from build123d import *

# Parameters (mm, degrees)
SKETCH1_R             = 45
SKETCH1_R_2           = 39
BOSS_EXTRUDE1_DEPTH   = 6
SKETCH1_R_3           = 8.5
BOSS_EXTRUDE1_2_DEPTH = 6
SKETCH4_R             = 39
SKETCH4_R_2           = 36
SKETCH4_R_3           = 11.5
SKETCH4_R_4           = 8.5
BOSS_EXTRUDE3_DEPTH   = 1.5
BOSS_EXTRUDE2_START   = -1.5
BOSS_EXTRUDE2_DEPTH   = 3
CIRPATTERN6_COUNT     = 6
FILLET1_R             = 3


# Read off the part's stored shape, not the designer's step: Boss-Extrude2
with BuildPart() as part:
    # Sketch1 → Boss-Extrude1 (new, symmetric)
    with BuildSketch(Plane.XY):
        Circle(SKETCH1_R)
        Circle(SKETCH1_R_2, mode=Mode.SUBTRACT)
    extrude(amount=BOSS_EXTRUDE1_DEPTH, both=True)



with BuildPart() as body_2:
    # Sketch1 → Boss-Extrude1 2 (new, symmetric)
    with BuildSketch(Plane.XY):
        Circle(SKETCH1_R_3)
        with BuildLine():
            Line((2, 1.5), (2, -1.5))
            ThreePointArc((2, -1.5), (-2.5, 0), (2, 1.5))
        make_face(mode=Mode.SUBTRACT)
    extrude(amount=BOSS_EXTRUDE1_2_DEPTH, both=True)


with BuildPart() as part_1:
    add(part.part)

    add(body_2.part)  # Boss-Extrude3 merges body 2
    # Sketch4 → Boss-Extrude3 (add, symmetric)
    # profile 1 of 2: a face of its own
    with BuildSketch(Plane.XY):
        Circle(SKETCH4_R)
        Circle(SKETCH4_R_2, mode=Mode.SUBTRACT)
    # profile 2 of 2: a face of its own
    with BuildSketch(Plane.XY):
        Circle(SKETCH4_R_3)
        Circle(SKETCH4_R_4, mode=Mode.SUBTRACT)
    extrude(amount=BOSS_EXTRUDE3_DEPTH, both=True)


with BuildPart() as body_2_2:
    # Boss-Extrude2 outline → Boss-Extrude2 (new body)
    with BuildSketch(Plane.XY.offset(BOSS_EXTRUDE2_START)):
        with BuildLine():
            Line((-4, 35.77708764), (-4, 10.781929326))
            ThreePointArc((-4, 10.781929326), (0, 11.5), (4, 10.781929326))
            Line((4, 10.781929326), (4, 35.77708764))
            ThreePointArc((4, 35.77708764), (0, 36), (-4, 35.77708764))
        make_face()
    extrude(amount=BOSS_EXTRUDE2_DEPTH)


with BuildPart() as cirpattern6_1:
    # CirPattern6: pattern copy
    add(body_2_2.part.rotate(Axis((0, 0, 0), (0, 0, 1)), 1 * 360 / CIRPATTERN6_COUNT))


with BuildPart() as cirpattern6_2:
    # CirPattern6: pattern copy
    add(body_2_2.part.rotate(Axis((0, 0, 0), (0, 0, 1)), 2 * 360 / CIRPATTERN6_COUNT))


with BuildPart() as cirpattern6_3:
    # CirPattern6: pattern copy
    add(body_2_2.part.rotate(Axis((0, 0, 0), (0, 0, 1)), 3 * 360 / CIRPATTERN6_COUNT))


with BuildPart() as cirpattern6_4:
    # CirPattern6: pattern copy
    add(body_2_2.part.rotate(Axis((0, 0, 0), (0, 0, 1)), 4 * 360 / CIRPATTERN6_COUNT))


with BuildPart() as cirpattern6_5:
    # CirPattern6: pattern copy
    add(body_2_2.part.rotate(Axis((0, 0, 0), (0, 0, 1)), 5 * 360 / CIRPATTERN6_COUNT))


with BuildPart() as part_2:
    add(part_1.part)

    # Combine1: union body 2 2, CirPattern6_5, CirPattern6_4, CirPattern6_3, CirPattern6_2, CirPattern6_1
    add(body_2_2.part)
    add(cirpattern6_5.part)
    add(cirpattern6_4.part)
    add(cirpattern6_3.part)
    add(cirpattern6_2.part)
    add(cirpattern6_1.part)

    # Fillet1
    fillet1_edges = [part_2.edges().sort_by_distance(p)[0] for p in [
        (-4, 10.781929326, 0),
        (-11.337424698, 1.926863048, 0),
        (-7.337424698, -8.855066278, 0),
        (4, -10.781929326, 0),
        (11.337424698, -1.926863048, 0),
        (7.337424698, 8.855066278, 0),
        (-4, 35.77708764, 0),
        (4, 10.781929326, 0),
        (4, 35.77708764, 0),
        (28.98386677, 21.352645435, 0),
        (11.337424698, 1.926863048, 0),
        (32.98386677, 14.424442205, 0),
        (32.98386677, -14.424442205, 0),
        (7.337424698, -8.855066278, 0),
        (28.98386677, -21.352645435, 0),
        (4, -35.77708764, 0),
        (-4, -10.781929326, 0),
        (-4, -35.77708764, 0),
        (-28.98386677, -21.352645435, 0),
        (-11.337424698, -1.926863048, 0),
        (-32.98386677, -14.424442205, 0),
        (-32.98386677, 14.424442205, 0),
        (-7.337424698, 8.855066278, 0),
        (-28.98386677, 21.352645435, 0),
    ]]
    fillet(fillet1_edges, radius=FILLET1_R)


solid = part_2.part
Read the model definition and answer for the solid it produces. Units are mm, in the model's axes. A direction names the side the tool comes from. Round coordinates to 2 decimals unless told otherwise and drop trailing zeros. Loops run counter-clockwise (first coordinate to the right, second up) from the corner with the lowest first, then second, coordinate; pieces in that order, holes last.
Q1. Section B-B on z = -4.5 is taken. Write down the section's boundary in (x, y).
Q2. Section C-C on x = -20 is taken. Write down the section's boundary in (y, z), and give its area (3 significant figures).
Q3. Section A-A on x = 0 is taken. Write down the section's boundary in (y, z), and give its area (3 significant figures).
Q4. Section D-D on x = 15.5 is taken. Write down the section's boundary in (y, z), and give its area (3 significant figures).
Q5. Consider probe 1 along Y at (x, z) = (0, 4.75); probe 2 along X at (y, z) = (15.5, -1); probe 3 along X at (y, z) = (-7.5, -2). Determine where each line is inside the solid, lowest interval first.
Q6. Determine the mould class of faces 4 (the face through (2, -2, -6)), 5 (the face through (-5.09, -34.56, 0.02)), 6 (the face through (36, 0, 0)) for opening direction Y: released by +Y, released by -Y, zero draft, split by the parting line, or undercut.
Q7. Which of the six approach directions +Z, -Z, +X, -X, +Y, -Y give full straight-line access (tool end or side, diameter ignored) to faces 1 (the face through (-1, 9, 1.5)), 2 (the face through (-1, 9, -1.5)), 3 (the face through (7.45, 9.41, 0.02))?
Q8. Each of these flat-tipped pins is pushed along its axis until it touches: pin 1 (4 mm diameter, centred on x = 12, z = 1.5, fed in from +Y); pin 2 (1.5 mm diameter, centred on x = 11, z = -2, fed in from -Y); pin 3 (6 mm diameter, centred on y = 12, z = 3, fed in from -X). Where does it stop, or does it pass through?
Output:
1. outline: circle Ø90 at (0, 0); circle Ø17 at (0, 0); hole circle Ø78 at (0, 0); hole (2, -1.5) - (2, 1.5) arc R2.5 ccw (long way) to start
2. outline: (-40.31, -6) - (-33.48, -6) - (-33.48, -1.5) - (-29.93, -1.5) - (-29.93, 1.5) - (-33.48, 1.5) - (-33.48, 6) - (-40.31, 6) - close; (-16.17, -1.5) - (-6.93, -1.5) - (-6.93, 1.5) - (-16.17, 1.5) - close; (6.93, -1.5) - (16.17, -1.5) - (16.17, 1.5) - (6.93, 1.5) - close; (29.93, -1.5) - (33.48, -1.5) - (33.48, -6) - (40.31, -6) - (40.31, 6) - (33.48, 6) - (33.48, 1.5) - (29.93, 1.5) - close
2. area: 241 mm2
3. outline: (-45, -6) - (-39, -6) - (-39, -1.5) - (-8.5, -1.5) - (-8.5, -6) - (-2.5, -6) - (-2.5, 6) - (-8.5, 6) - (-8.5, 1.5) - (-39, 1.5) - (-39, 6) - (-45, 6) - close; (2.5, -6) - (8.5, -6) - (8.5, -1.5) - (39, -1.5) - (39, -6) - (45, -6) - (45, 6) - (39, 6) - (39, 1.5) - (8.5, 1.5) - (8.5, 6) - (2.5, 6) - close
3. area: 471 mm2
4. outline: (-42.25, -6) - (-35.79, -6) - (-35.79, -1.5) - (-32.49, -1.5) - (-32.49, 1.5) - (-35.79, 1.5) - (-35.79, 6) - (-42.25, 6) - close; (-13.57, -1.5) - (-4.33, -1.5) - (-4.33, 1.5) - (-13.57, 1.5) - close; (4.33, -1.5) - (13.57, -1.5) - (13.57, 1.5) - (4.33, 1.5) - close; (32.49, -1.5) - (35.79, -1.5) - (35.79, -6) - (42.25, -6) - (42.25, 6) - (35.79, 6) - (35.79, 1.5) - (32.49, 1.5) - close
4. area: 230 mm2
5. probe 1: y = -45 to -39, -8.5 to -2.5, 2.5 to 8.5, 39 to 45
5. probe 2: x = -42.25 to -18.85, -4 to 4, 18.85 to 42.25
5. probe 3: x = -44.37 to -38.27, -4 to 4, 38.27 to 44.37
6. face 4: zero draft
6. face 5: undercut
6. face 6: undercut
7. face 1: +Z
7. face 2: -Z
7. face 3: +Z, -Z
8. pin 1: stops at y = 43.87
8. pin 2: stops at y = -43.82
8. pin 3: stops at x = -44.09
